The model under review builds one solid part; all positions refer to its coordinate system, in mm. A direction names the side the tool comes from. Give positions to 0.01 mm unless a question says otherwise; leave off trailing zeros. Order: outer loops, then holes, each group sorted by start corner. A loop starts at its lowest first (then second) coordinate and runs counter-clockwise, first axis right, second up. Notation, with made-up numbers: (-19.5, 82.5) -> (2.5, 82.5) arc R25 cw to (2.5, 105.5) -> close; hole circle Ø11 at (16.5, 9). An arc over 180 degrees is marked (long way). Use one line per item in the form item = value.
```python
from build123d import *

# Parameters (mm, degrees)
EXTRUDE_1_DEPTH          = 12.75
EXTRUDE_1_DEPTH_BACK     = 12.75
EXTRUDE_1_2_DEPTH        = 1.2
EXTRUDE_2_DEPTH          = 1.2
SKETCH_4_W               = 23.6
SKETCH_4_H               = 23.6
CUT_EXTRUDE_1_DEPTH      = 1.5
CUT_EXTRUDE_2_DEPTH      = 35.680906203
CUT_EXTRUDE_2_DEPTH_BACK = 35.680906203
SKETCH_5_W               = 13.95
SKETCH_5_H               = 32.801494515
EXTRUDE_3_DEPTH          = 3


with BuildPart() as part:
    # Эскиз1 → Extrude 1 (new, two sides: drawn at the far end of the back side and taken through both)
    with BuildSketch(Plane.XY.offset(-EXTRUDE_1_DEPTH_BACK)):
        Polygon((-17.621320344, -13.5), (17.621320344, -13.5), (25.211407429, -5.909912914), (0, 19.301494515), (-25.211407429, -5.909912914), align=None)
        Polygon((-17, -12), (17, -12), (23.090087086, -5.909912914), (0, 17.180174171), (-23.090087086, -5.909912914), align=None, mode=Mode.SUBTRACT)
    extrude(amount=EXTRUDE_1_DEPTH + EXTRUDE_1_DEPTH_BACK)

    # Эскиз2 → Extrude 1 2 (add)
    with BuildSketch(Plane.XY.offset(12.75)):
        Polygon((25.211407429, -5.909912914), (0, 19.301494515), (-25.211407429, -5.909912914), (-17.621320344, -13.5), (17.621320344, -13.5), align=None)
    extrude(amount=EXTRUDE_1_2_DEPTH)

    # Эскиз3 → Бобышка-Вытянуть2 (add)
    with BuildSketch(Plane(origin=(0, 0, -12.75), x_dir=(-1, 0, 0), z_dir=(0, 0, -1))):
        Polygon((0, 19.301494515), (25.211407429, -5.909912914), (17.621320344, -13.5), (-17.621320344, -13.5), (-25.211407429, -5.909912914), align=None)
    extrude(amount=EXTRUDE_2_DEPTH)

    # Эскиз4 → Вырез-Вытянуть1 (cut)
    with BuildSketch(Plane.XZ.offset(13.5)):
        Rectangle(SKETCH_4_W, SKETCH_4_H)
    extrude(amount=-CUT_EXTRUDE_1_DEPTH, mode=Mode.SUBTRACT)

    # Эскиз5 → Вырез-Вытянуть2 (cut, two sides: drawn at the far end of the back side and taken through both)
    with BuildSketch(Plane(origin=(0, 0, 0), x_dir=(0, 0, -1), z_dir=(1, 0, 0)).offset(-CUT_EXTRUDE_2_DEPTH_BACK)):
        with Locations((6.975, 2.900747258)):
            Rectangle(SKETCH_5_W, SKETCH_5_H)
    extrude(amount=CUT_EXTRUDE_2_DEPTH + CUT_EXTRUDE_2_DEPTH_BACK, mode=Mode.SUBTRACT)

    # Эскиз7 → Бобышка-Вытянуть3 (add)
    with BuildSketch(Plane(origin=(0, 0, 0), x_dir=(-1, 0, 0), z_dir=(0, 0, -1))):
        Polygon((-17.289949494, -12.7), (-11.8, -12.7), (-11.8, -12), (-17, -12), (-23.090087086, -5.909912914), (0, 17.180174171), (23.090087086, -5.909912914), (17, -12), (11.8, -12), (11.8, -12.7), (17.289949494, -12.7), (24.080036579, -5.909912914), (0, 18.170123665), (-24.080036579, -5.909912914), align=None)
    extrude(amount=EXTRUDE_3_DEPTH)


solid = part.part
```
1. The part is to be moulded in two halves that separate along X. For faces 6 (the face through (11, 8, 0)), 7 (the face through (-12.21, 5.96, -1.48)), 8 (the face through (0, 0, 12.75)), say which applies: +X half, -X half, draft (parallel to the pull), parting line (faces both ways), or undercut.
Values:
face_6 = draft
face_7 = -X half
face_8 = undercut
2. Add section C-C on x = -8.5. Give the boundary of the cut face in (y, z).
Values:
outline = (-13.5, 11.8) -> (-12, 11.8) -> (-12, 12.75) -> (8.68, 12.75) -> (8.68, -3) -> (9.67, -3) -> (9.67, 0) -> (10.8, 0) -> (10.8, 13.95) -> (-13.5, 13.95) -> close
3. For L1, parallel to X at y = 16.5, z = 11.75; L2, parallel to X at y = 1, z = 6.75; L3, parallel to Z at x = -18, y = -2.5, list the stretches that pass through material, from the lowest coordinate up.
Values:
L1 = -2.8 to -0.68, 0.68 to 2.8
L2 = -18.3 to -16.18, 16.18 to 18.3
L3 = 12.75 to 13.95
4. Tool access review of faces 1 (the face through (11.8, -13, 5)), 2 (the face through (11.87, 6.3, -1.48)), 3 (the face through (15, -12.7, -1)), 4 (the face through (-3, -12, 12)), 5 (the face through (20.73, -9.26, -1.48)): name each direction out of +Z, -Z, +X, -X, +Y, -Y from which nothing blocks a thin tool from reaching the whole face with its end or side.
Values:
face_1 = -Z, -Y
face_2 = -Z, +X, +Y
face_3 = -Z, +X, -X, -Y
face_4 = -Z
face_5 = -Z, +X, -Y
5. Add section D-D on y = 15.5. Give the boundary of the cut face in (x, z).
Values:
outline = (-3.8, 0) -> (-2.67, 0) -> (-2.67, -3) -> (-1.68, -3) -> (-1.68, 12.75) -> (1.68, 12.75) -> (1.68, -3) -> (2.67, -3) -> (2.67, 0) -> (3.8, 0) -> (3.8, 13.95) -> (-3.8, 13.95) -> close
6. Add section A-A on z = -1.5. Give the boundary of the cut face in (x, y), then the cut area to 3 significant figures.
Values:
outline = (-24.08, -5.91) -> (-17.29, -12.7) -> (-11.8, -12.7) -> (-11.8, -12) -> (-17, -12) -> (-23.09, -5.91) -> (0, 17.18) -> (23.09, -5.91) -> (17, -12) -> (11.8, -12) -> (11.8, -12.7) -> (17.29, -12.7) -> (24.08, -5.91) -> (0, 18.17) -> close
area = 66.9 mm^2
7. Add section B-B on y = -3. Give the boundary of the cut face in (x, z), then the cut area to 3 significant figures.
Values:
outline = (-22.3, 0) -> (-21.17, 0) -> (-21.17, -3) -> (-20.18, -3) -> (-20.18, 12.75) -> (20.18, 12.75) -> (20.18, -3) -> (21.17, -3) -> (21.17, 0) -> (22.3, 0) -> (22.3, 13.95) -> (-22.3, 13.95) -> close
area = 114 mm^2
8. For pin 1 Ø1.6 at (y, z) = (-13, 3) entering from -X; pin 2 Ø10 at (x, y) = (-12.5, 10.5) entering from -Z; pin 3 Ø8 at (x, z) = (11, 12) entering from +Y; pin 4 Ø1.5 at (y, z) = (8.5, -0.5) entering from -X, all flat-tipped, find the tip position at first contact; note any pin that passes through.
Values:
pin_1 = -18.92
pin_2 = -3
pin_3 = 12.3
pin_4 = -11.36
